Design review of the part built by this model. Coordinates are the model's own, in mm. A direction names the side the tool comes from. Round coordinates to 2 decimals unless told otherwise and drop trailing zeros. Write each loop counter-clockwise with the first axis right and the second up, starting at its lowest first coordinate (ties: lowest second). Pieces come first, ordered by that corner, then holes. Notation, with made-up numbers: (59.5, 22) -> (73.5, 22) arc R14 ccw to (73.5, 47) -> close; hole circle Ø5 at (30.5, 17). An arc over 180 degrees is marked (long way). One line per question, with ' | ' between items. Start each with the question number.
1) For probe 1 along Y at (x, z) = (20, 28); probe 2 along Y at (x, z) = (34, 13); probe 3 along X at (y, z) = (60, 16), list the stretches that pass through material, from the lowest coordinate up.
2) Consider section A-A (y = 57). Give the boundary of the cut face in (x, z).
3) Consider section C-C (y = 72). Give the boundary of the cut face in (x, z).
4) Mouldability with a two-part tool opening along Z and no side actions: class faces 1 (the flat face through (20, 41, 0)), 2 (the cylindrical face through (35.144, 81.974, 12.328)), 3 (the flat face through (30.15, 73, 13)) as +Z half, -Z half, draft (parallel to the pull), parting line (faces both ways), or undercut.
5) Insertion check: pin 1 Ø4.5 at (x, y) = (20, 85) entering from -Z; pin 2 Ø7.5 at (x, y) = (20, 25.15) entering from -Z; pin 3 Ø10 at (x, z) = (18.5, 8.5) entering from +Y; pin 4 Ø16 at (x, y) = (20, 28.5) entering from -Z. Each pin has a flat end and moves straight along its axis. Give the tip position at first contact, or say it passes through.
6) Consider section B-B (z = 13). Count the separate pieces of the cut face and the enclosed holes in it, then the cut area to 3 significant figures.
7) For faces 4 (the flat face through (20, 73, 23)), 5 (the flat face through (20, 29, 25)), 6 (the cylindrical face through (39.1, 99.14, 16.27)), list the 3-axis set-ups (+Z, -Z, +X, -X, +Y, -Y) from which the entire face can be reached by the end or side of a thin tool; tool diameter is ignored.
```python
from build123d import *

# Parameters (mm, degrees)
SKETCH1_W               = 40
SKETCH1_H               = 100
BOSS_EXTRUDE1_DEPTH     = 25
BOSS_EXTRUDE2_START     = 25
SKETCH1_3_W             = 40
SKETCH1_3_H             = 100
SKETCH1_3_R             = 2.75
BOSS_EXTRUDE2_DEPTH     = 8
CUT_EXTRUDE1_START      = -50
SKETCH2_W               = 20.3
SKETCH2_H               = 23
CUT_EXTRUDE1_DEPTH      = 63.645461515
CUT_EXTRUDE2_DEPTH      = 110.535485118
CUT_EXTRUDE2_DEPTH_BACK = 110.535485118
SKETCH3_R               = 3.1
SKETCH4_R               = 2.75
CUT_EXTRUDE3_DEPTH      = 111.131739294
FILLET1_R               = 3
FILLET2_R               = 1
SKETCH6_R               = 3.25
CUT_EXTRUDE4_DEPTH      = 111.56672196


with BuildPart() as part:
    # Sketch1 → Boss-Extrude1 (new body)
    with BuildSketch(Plane.XY):
        with Locations((20, 50)):
            Rectangle(SKETCH1_W, SKETCH1_H)
        with BuildLine():
            Line((22.975, 37.8), (22.975, 34.854219443))
            ThreePointArc((22.975, 34.854219443), (28.161456671, 31.184328877), (30.15, 25.15))
            ThreePointArc((30.15, 25.15), (13.965671123, 16.988543329), (17.025, 34.854219443))
            Line((17.025, 34.854219443), (17.025, 37.8))
            Line((17.025, 37.8), (22.975, 37.8))
        make_face(mode=Mode.SUBTRACT)
    extrude(amount=BOSS_EXTRUDE1_DEPTH)

    # Sketch1<3> → Boss-Extrude2 (add)
    with BuildSketch(Plane.XY.offset(BOSS_EXTRUDE2_START)):
        with Locations((20, 50)):
            Rectangle(SKETCH1_3_W, SKETCH1_3_H)
        with Locations((20, 25.15)):
            Circle(SKETCH1_3_R, mode=Mode.SUBTRACT)
    extrude(amount=BOSS_EXTRUDE2_DEPTH)

    # Sketch2 → Cut-Extrude1 (cut, through all)
    with BuildSketch(Plane.XZ.offset(CUT_EXTRUDE1_START)):
        with Locations((20, 11.5)):
            Rectangle(SKETCH2_W, SKETCH2_H)
    extrude(amount=-CUT_EXTRUDE1_DEPTH, mode=Mode.SUBTRACT)

    # Sketch3 → Cut-Extrude2 (cut, two sides: drawn at the far end of the back side and taken through both)
    with BuildSketch(Plane.ZY.offset(-30.15).offset(-CUT_EXTRUDE2_DEPTH_BACK)):
        with Locations((13, 57)):
            Circle(SKETCH3_R)
        with Locations((13, 85)):
            Circle(SKETCH3_R)
    extrude(amount=CUT_EXTRUDE2_DEPTH + CUT_EXTRUDE2_DEPTH_BACK, mode=Mode.SUBTRACT)

    # Sketch4 → Cut-Extrude3 (cut, through all)
    with BuildSketch(Plane(origin=(0, 0, 23), x_dir=(-1, 0, 0), z_dir=(0, 0, -1))):
        with Locations((-20, 57)):
            Circle(SKETCH4_R)
        with Locations((-20, 85)):
            Circle(SKETCH4_R)
    extrude(amount=-CUT_EXTRUDE3_DEPTH, mode=Mode.SUBTRACT)

    # Fillet1
    fillet1_edges = [part.edges().sort_by_distance(p)[0] for p in [
        (0, 50, 0),
        (40, 50, 0),
        (20, 0, 0),
        (0, 0, 16.5),
        (0, 100, 16.5),
        (40, 100, 16.5),
        (40, 0, 16.5),
        (9.85, 100, 11.5),
        (9.85, 75, 0),
        (20, 100, 23),
        (30.15, 100, 11.5),
        (30.15, 75, 0),
        (20, 50, 0),
    ]]
    fillet(fillet1_edges, radius=FILLET1_R)

    # Fillet2
    fillet2_edges = [part.edges().sort_by_distance(p)[0] for p in [
        (22.975, 36.327109722, 0),
        (20, 37.8, 0),
        (17.025, 36.327109722, 0),
        (20, 15, 0),
    ]]
    fillet(fillet2_edges, radius=FILLET2_R)

    # Sketch6 → Cut-Extrude4 (cut, through all)
    with BuildSketch(Plane(origin=(0, 0, 25), x_dir=(-1, 0, 0), z_dir=(0, 0, -1))):
        with Locations((-20, 25.15)):
            Circle(SKETCH6_R)
    extrude(amount=-CUT_EXTRUDE4_DEPTH, mode=Mode.SUBTRACT)


solid = part.part
```
From the geometry:
1) probe 1: y = 0 to 21.9, 28.4 to 54.25, 59.75 to 82.25, 87.75 to 100 | probe 2: y = 0 to 53.9, 60.1 to 81.9, 88.1 to 100 | probe 3: x = 0 to 9.85, 30.15 to 40
2) outline: (0, 3) arc R3 ccw to (3, 0) -> (6.85, 0) arc R3 ccw to (9.85, 3) -> (9.85, 9.9) -> (0, 9.9) -> close; (0, 16.1) -> (9.85, 16.1) -> (9.85, 23) -> (17.25, 23) -> (17.25, 33) -> (0, 33) -> close; (22.75, 23) -> (30.15, 23) -> (30.15, 16.1) -> (40, 16.1) -> (40, 33) -> (22.75, 33) -> close; (30.15, 3) arc R3 ccw to (33.15, 0) -> (37, 0) arc R3 ccw to (40, 3) -> (40, 9.9) -> (30.15, 9.9) -> close
3) outline: (0, 3) arc R3 ccw to (3, 0) -> (6.85, 0) arc R3 ccw to (9.85, 3) -> (9.85, 23) -> (30.15, 23) -> (30.15, 3) arc R3 ccw to (33.15, 0) -> (37, 0) arc R3 ccw to (40, 3) -> (40, 33) -> (0, 33) -> close
4) face 1: -Z half | face 2: undercut | face 3: draft
5) pin 1: passes through | pin 2: stops at z = 25 | pin 3: stops at y = 50 | pin 4: stops at z = 0
6) separate pieces: 5 | enclosed holes: 1 | area: 2,390 mm2
7) face 4: -Z, +Y | face 5: -Z | face 6: +Z, -Z, +X, +Y
